```python
from build123d import *

# Parameters (mm, degrees)
SKETCH1_R           = 7.7
BOSS_EXTRUDE1_DEPTH = 6
CHAMFER1_SIZE       = 2
SKETCH4_W           = 8
SKETCH4_H           = 45.5
SKETCH4_R           = 2
BOSS_EXTRUDE2_DEPTH = 3
CHAMFER2_SIZE       = 2


with BuildPart() as part:
    # Sketch1 → Boss-Extrude1 (new body)
    with BuildSketch(Plane(origin=(0, 0, 0), x_dir=(0, 0, -1), z_dir=(1, 0, 0))):
        with BuildLine():
            Line((0, 13.7), (39, 13.7))
            Line((39, 13.7), (39, -13.7))
            Line((39, -13.7), (0, -13.7))
            ThreePointArc((0, -13.7), (-13.7, 0), (0, 13.7))
        make_face()
        Circle(SKETCH1_R, mode=Mode.SUBTRACT)
        with BuildLine():
            Line((11.331372379, 7.7), (33, 7.7))
            Line((33, 7.7), (33, -7.7))
            Line((33, -7.7), (11.331372379, -7.7))
            ThreePointArc((11.331372379, -7.7), (13.7, 0), (11.331372379, 7.7))
        make_face(mode=Mode.SUBTRACT)
    extrude(amount=BOSS_EXTRUDE1_DEPTH)

    # Chamfer1
    chamfer1_edges = [part.edges().sort_by_distance(p)[0] for p in [
        (6, 13.7, -19.5),
        (0, 0, -33),
        (0, 7.7, -22.16568619),
        (0, 0, -13.7),
        (0, -7.7, -22.16568619),
        (6, 0, -33),
        (6, 7.7, -22.16568619),
        (6, 0, -13.7),
        (6, -7.7, -22.16568619),
        (0, 0, 7.7),
        (6, 0, 7.7),
        (6, 0, 13.7),
        (0, 13.7, -19.5),
        (0, -13.7, -19.5),
        (0, 0, 13.7),
        (6, -13.7, -19.5),
    ]]
    chamfer(chamfer1_edges, length=CHAMFER1_SIZE)

    # Sketch4 → Boss-Extrude2 (add)
    with BuildSketch(Plane(origin=(0, 0, -39), x_dir=(-1, 0, 0), z_dir=(0, 0, -1))):
        with Locations((-2, 0)):
            Rectangle(SKETCH4_W, SKETCH4_H)
        with Locations((-2, 18.75)):
            Circle(SKETCH4_R, mode=Mode.SUBTRACT)
        with Locations(Location((-2, -18.75, 0), (0, 0, 180))):
            Circle(SKETCH4_R, mode=Mode.SUBTRACT)
    extrude(amount=BOSS_EXTRUDE2_DEPTH)

    # Chamfer2
    chamfer2_edges = [part.edges().sort_by_distance(p)[0] for p in [
        (6, -22.75, -40.5),
        (-2, -22.75, -40.5),
        (6, 22.75, -40.5),
        (-2, 22.75, -40.5),
    ]]
    chamfer(chamfer2_edges, length=CHAMFER2_SIZE)


solid = part.part
```
Source: CAD feature listing. Evaluate the final solid. Frame: model axes, mm. A direction names the side the tool comes from. Coordinates: 2 decimals unless noted, no trailing zeros. Order: outer loops, then holes, each group sorted by start corner. A loop starts at its lowest first (then second) coordinate and runs counter-clockwise, first axis right, second up. Notation, with made-up numbers: (14, 54) - (72, 54) arc R20 cw to (72, 65) - close; hole circle Ø9 at (87.5, 2.25). An arc over 180 degrees is marked (long way). One line per item, written item: value.
1) Cut plane C-C on z = -16. Output: boundary loops of the cut face in (x, y).
Computed values:
outline: (0, -11.7) - (2, -13.7) - (4, -13.7) - (6, -11.7) - (6, -9.7) - (4, -7.7) - (2, -7.7) - (0, -9.7) - close; (0, 9.7) - (2, 7.7) - (4, 7.7) - (6, 9.7) - (6, 11.7) - (4, 13.7) - (2, 13.7) - (0, 11.7) - close
2) Cut plane D-D on y = -18.75. Output: boundary loops of the cut face in (x, z).
Computed values:
outline: (-2, -42) - (0, -42) - (0, -39) - (-2, -39) - close; (4, -42) - (6, -42) - (6, -39) - (4, -39) - close
3) Contact query for flat-ended pins moving along their axis: pin 1 (4 mm diameter, centred on x = 4.5, y = -13, fed in from +Z); pin 2 (0.6 mm diameter, centred on x = 2.5, z = -24, fed in from +Y); pin 3 (12 mm diameter, centred on y = 1.5, z = -29.5, fed in from -X). Output: stop coordinate, or through.
Computed values:
pin 1: stops at z = 8.08
pin 2: stops at y = 13.7
pin 3: stops at x = 0
4) Reachability of faces 1 (the face through (0.3, -0.2, -12)), 2 (the face through (1, 12.7, -19.2)), 3 (the face through (5, 12.7, -19.2)), 4 (the face through (5, -8.7, -21)) from +Z, -Z, +X, -X, +Y, -Y: full face, straight path, thin tool, end or side. Return the list, or none.
Computed values:
face 1: -X
face 2: +Z, -X, +Y
face 3: +Z, +X, +Y
face 4: +X
5) Ray query, line 1 (Y direction, x = 2, z = -39.7); line 2 (Z direction, x = 5, y = -4.5); line 3 (Z direction, x = 2.25, y = 2.5). Return the intervals inside material, ascending. Write a range as [from, to].
Computed values:
line 1: y = [-22.75, -20.75], [-16.75, 16.75], [20.75, 22.75]
line 2: z = [-42, -34], [-11.88, -7.45], [7.45, 11.88]
line 3: z = [-42, -33], [-13.47, -7.28], [7.28, 13.47]
6) Cut plane B-B on x = 1. Output: boundary loops of the cut face in (y, z), plus the area to 3 significant figures.
Computed values:
outline: (-22.75, -42) - (-20.48, -42) - (-20.48, -39) - (-22.75, -39) - close; (-17.02, -42) - (17.02, -42) - (17.02, -39) - (12.7, -39) - (12.7, 0) arc R12.7 ccw to (-12.7, 0) - (-12.7, -39) - (-17.02, -39) - close; (20.48, -42) - (22.75, -42) - (22.75, -39) - (20.48, -39) - close; hole (-8.7, -34) - (8.7, -34) - (8.7, -9.25) arc R12.7 cw to (-8.7, -9.25) - close; hole circle Ø17.4 at (0, 0)
area: 732 mm^2
7) Cut plane A-A on y = 0. Output: boundary loops of the cut face in (x, z), plus the area to 3 significant figures.
Computed values:
outline: (-2, -42) - (6, -42) - (6, -35) - (4, -33) - (2, -33) - (0, -35) - (0, -39) - (-2, -39) - close; (0, -11.7) - (2, -13.7) - (4, -13.7) - (6, -11.7) - (6, -9.7) - (4, -7.7) - (2, -7.7) - (0, -9.7) - close; (0, 9.7) - (2, 7.7) - (4, 7.7) - (6, 9.7) - (6, 11.7) - (4, 13.7) - (2, 13.7) - (0, 11.7) - close
area: 112 mm^2
8) Mould query, pull axis Z, two halves, no side actions, for faces 5 (the face through (0.32, -0.26, 12.02)), 6 (the face through (5, 0, -34)), 7 (the face through (2, 22.75, -40)). Classes: released by +Z, released by -Z, zero draft, split by the parting line, or undercut.
Computed values:
face 5: released by +Z
face 6: undercut
face 7: zero draft
